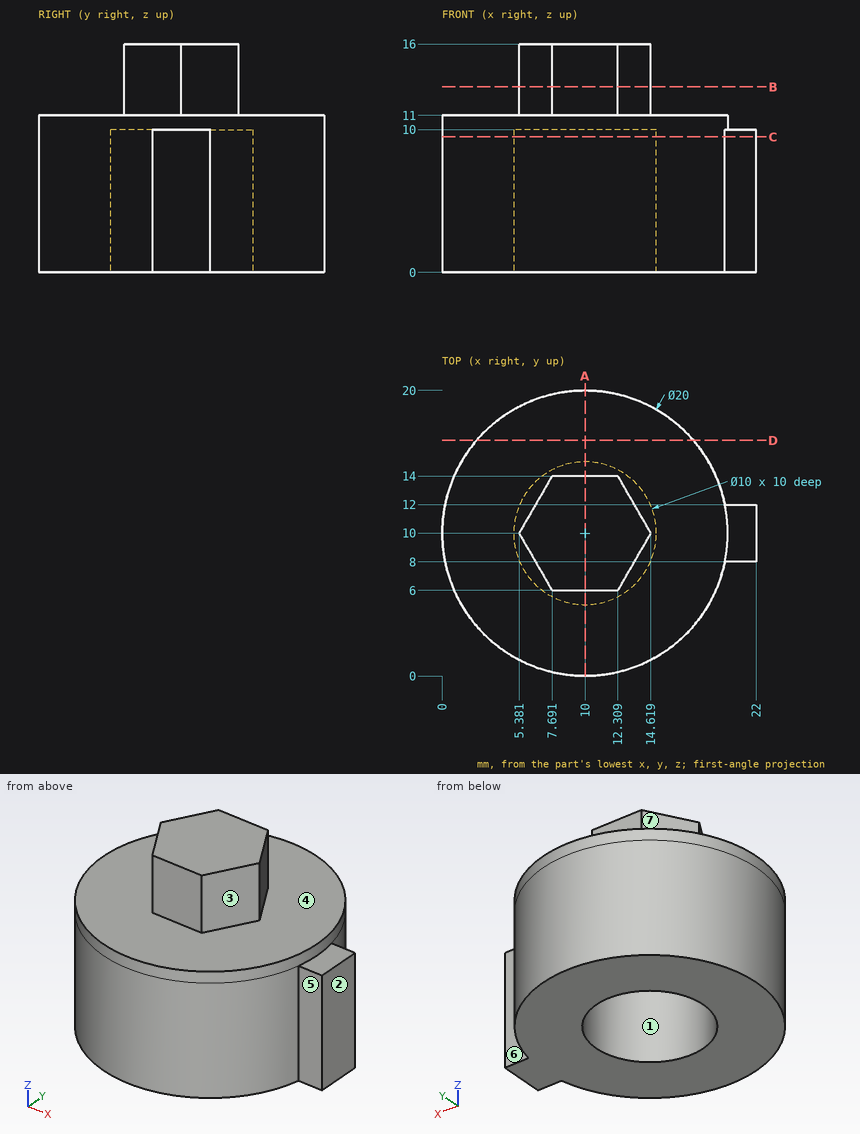
Geometry: see drawing. Coordinates: mm, zero at the bounding-box minimum. A direction names the side the tool comes from. Round coordinates to 2 decimals unless told otherwise and drop trailing zeros. Write each loop counter-clockwise with the first axis right and the second up, starting at its lowest first coordinate (ties: lowest second). Pieces come first, ordered by that corner, then holes. Notation, with made-up numbers: (4, 35.5) - (35, 35.5) arc R17 ccw to (35, 53.5) - close; hole circle Ø10 at (85.5, 10.25). An arc over 180 degrees is marked (long way). Use CSV: the item, a comma, the result in double quotes. Start each with the question number.
(1) Cut plane C-C, the plane z = 9.5. Return loops of the section in (x, y).
(2) Material intervals for probe 1 along Y at (x, z) = (10, 4); probe 2 along X at (y, z) = (9.75, 9); probe 3 along Z at (x, y) = (10.5, 16.25), sorted ascending. Write a range as [from, to].
(3) Cut plane B-B, the plane z = 13. Return loops of the section in (x, y).
(4) First-contact query: pin 1 Ø3.5 at (x, z) = (9.5, 14) entering from -Y; pin 2 Ø2 at (y, z) = (13.5, 5.5) entering from +X; pin 3 Ø6 at (x, y) = (17.5, 11.5) entering from +Z; pin 4 Ø8 at (y, z) = (12, 11.5) entering from +X. Flat tips, straight axial feed; report the tip coordinate or a pass-through.
(5) Mould query, pull axis Y, two halves, no side actions, for the marked faces 1, 2 and 3. Classes: pulls with the +Y half, pulls with the -Y half, needs draft (parallel to the pull), parting line crosses it, or undercut.
(6) Cut plane D-D, the plane y = 16.5. Return loops of the section in (x, z).
(7) Cut plane A-A, the plane x = 10. Return loops of the section in (y, z).
(8) Set-up query: the marked faces 4, 5, 6 and 7. Return all of +Z, -Z, +X, -X, +Y, -Y with unobstructed straight access to the full face (end or side cutting, diameter ignored); none if empty.
Geometry says:
1,outline,"(19.8, 8) - (22, 8) - (22, 12) - (19.8, 12) arc R10 ccw (long way) to start; hole circle Ø10 at (10, 10)"
2,probe 1,"[0, 5], [15, 20]"
2,probe 2,"[0, 5.01], [14.99, 22]"
2,probe 3,"[0, 11]"
3,outline,"(5.38, 10) - (7.69, 6) - (12.31, 6) - (14.62, 10) - (12.31, 14) - (7.69, 14) - close"
4,pin 1,"y = 6"
4,pin 2,"x = 19.68"
4,pin 3,"z = 11"
4,pin 4,"x = 22"
5,face 1,"undercut"
5,face 2,"needs draft"
5,face 3,"pulls with the -Y half"
6,outline,"(2.4, 0) - (17.6, 0) - (17.6, 11) - (2.4, 11) - close"
7,outline,"(0, 0) - (5, 0) - (5, 10) - (15, 10) - (15, 0) - (20, 0) - (20, 11) - (14, 11) - (14, 16) - (6, 16) - (6, 11) - (0, 11) - close"
8,face 4,"+Z"
8,face 5,"+Z, -Z, +X, -Y"
8,face 6,"+Z, -Z, +X, +Y"
8,face 7,"+Z, -X, +Y"
